Here's the drawing with two shaded views (mm, measured from the low corner). I have some questions. A direction names the side the tool comes from. Give positions to 0.01 mm unless a question says otherwise; leave off trailing zeros. Loops run counter-clockwise (first coordinate to the right, second up) from the corner with the lowest first, then second, coordinate; pieces in that order, holes last.
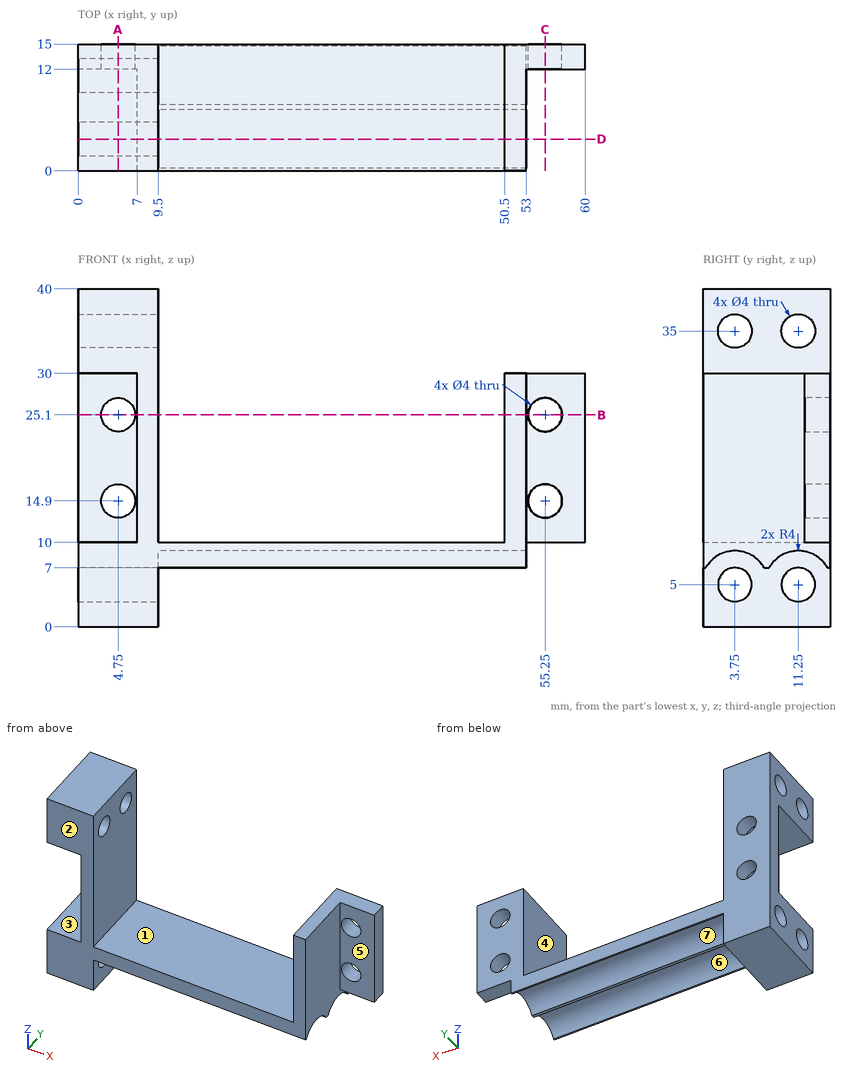
(1) Please list where these lines run through material, in increasing order: probe 1 along Y at (x, z) = (2, 35); probe 2 along Z at (x, y) = (55.25, 13.35); probe 3 along X at (y, z) = (4.5, 17).
Returned:
probe 1: y = 0 to 1.75, 5.75 to 9.25, 13.25 to 15
probe 2: z = 10 to 12.9, 16.9 to 23.1, 27.1 to 30
probe 3: x = 7 to 9.5, 50.5 to 53
(2) Suppose I cut it at A-A on x = 4.75. List the corners of the cut face in (y, z) for me, plus the area to 3 significant figures.
Returned:
outline: (0, 0) - (15, 0) - (15, 12.9) - (12, 12.9) - (12, 10) - (0, 10) - close; (0, 30) - (12, 30) - (12, 27.1) - (15, 27.1) - (15, 40) - (0, 40) - close; (12, 16.9) - (15, 16.9) - (15, 23.1) - (12, 23.1) - close; hole circle Ø4 at (3.75, 5); hole circle Ø4 at (3.75, 35); hole circle Ø4 at (11.25, 5); hole circle Ø4 at (11.25, 35)
area: 286 mm2
(3) Suppose I cut it at D-D on y = 3.75. List the corners of the cut face in (x, z) for me.
Returned:
outline: (0, 0) - (9.5, 0) - (9.5, 3) - (0, 3) - close; (0, 7) - (9.5, 7) - (9.5, 9) - (53, 9) - (53, 30) - (50.5, 30) - (50.5, 10) - (9.5, 10) - (9.5, 33) - (0, 33) - (0, 30) - (7, 30) - (7, 10) - (0, 10) - close; (0, 37) - (9.5, 37) - (9.5, 40) - (0, 40) - close
(4) Thinking about a two-plate mould opening in Y: for the marked faces 4, 5, 6 and 7, which applies, pulls with the +Y half, pulls with the -Y half, needs draft (parallel to the pull), parting line crosses it, or undercut?
Returned:
face 4: needs draft
face 5: pulls with the -Y half
face 6: undercut
face 7: undercut
(5) Which directions (+Z, -Z, +X, -X, +Y, -Y) give clear straight access to the entire face, cutting with the end or side of a thin tool? Please do the marked faces 1, 2 and 3.
Returned:
face 1: +Z, +Y, -Y
face 2: +Z, -Z, +X, -X, -Y
face 3: -X, -Y
(6) Suppose I cut it at B-B on z = 25.1. List the corners of the cut face in (x, y) for me, plus the area to 3 significant figures.
Returned:
outline: (0, 12) - (2.75, 12) - (2.75, 15) - (0, 15) - close; (6.75, 12) - (7, 12) - (7, 0) - (9.5, 0) - (9.5, 15) - (6.75, 15) - close; (50.5, 0) - (53, 0) - (53, 12) - (53.25, 12) - (53.25, 15) - (50.5, 15) - close; (57.25, 12) - (60, 12) - (60, 15) - (57.25, 15) - close
area: 93.0 mm2
(7) Suppose I cut it at C-C on x = 55.25. List the corners of the cut face in (y, z) for me, plus the area to 3 significant figures.
Returned:
outline: (12, 10) - (15, 10) - (15, 12.9) - (12, 12.9) - close; (12, 16.9) - (15, 16.9) - (15, 23.1) - (12, 23.1) - close; (12, 27.1) - (15, 27.1) - (15, 30) - (12, 30) - close
area: 36.0 mm2
(8) Will these pins go through, and if not, where does the flat tip stop? P1, Ø8, axis at x = 26, z = 5.5, coming from the +Y side; P2, Ø2, axis at x = 42.5, y = 12, coming from the -Z side; P3, Ø2.5, axis at x = 55.25, z = 25.1, coming from the +Y side; P4, Ø1.5, axis at x = 38, y = 7, coming from the +Z side.
Returned:
P1: stops at y = 15
P2: stops at z = 8.6
P3: passes through
P4: stops at z = 10
